Source: CAD feature listing. Evaluate the final solid. Frame: model axes, mm. Give positions to 0.01 mm unless a question says otherwise; leave off trailing zeros. Loops run counter-clockwise (first coordinate to the right, second up) from the corner with the lowest first, then second, coordinate; pieces in that order, holes last. Notation, with made-up numbers: (-39.5, 35.25) -> (-30.5, 35.25) arc R33 cw to (-30.5, 71.25) -> close; hole circle Ø5 at (84, -29.75). An arc over 180 degrees is marked (long way). Return JSON: item names as keys, results as strings. Group by question number.
(1) Cut plane C-C on z = -23. Return loops of the section in (x, y), then the cut area to 3 significant figures.
(2) Ray query, line 1 (X direction, y = 3.5, z = -107); line 2 (X direction, y = 0.5, z = 9). Return the intervals inside material, ascending. Write a range as from..to.
(3) Cut plane B-B on y = 0.5. Give the number of separate pieces and of enclosed holes in the cut face, then the cut area to 3 significant figures.
(4) Cut plane A-A on z = 104.5. Return loops of the section in (x, y).
(5) Pin query (flat end, axial travel): pin 1 (2.5 mm diameter, centred on x = -520, y = 0.5, fed in from -Z); pin 2 (2.5 mm diameter, centred on y = -0.5, z = -11, fed in from +X); pin 3 (2.5 mm diameter, centred on x = 528, y = 1, fed in from +Z). Return the tip coordinate at first contact, or that it passes through.
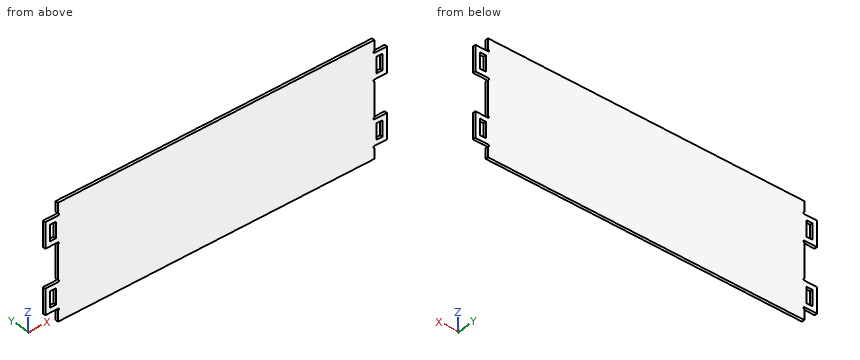
```python
from build123d import *

# Parameters (mm, degrees)
SKETCH1_W           = 18
SKETCH1_H           = 50
BOSS_EXTRUDE1_DEPTH = 4.3


with BuildPart() as part:
    # Sketch1 → Boss-Extrude1 (new body, symmetric)
    with BuildSketch(Plane(origin=(0, 0, 0), x_dir=(1, 0, 0), z_dir=(0, 1, 0))):
        with BuildLine():
            Line((-500, 179), (500, 179))
            Line((500, 179), (500, 146.36))
            ThreePointArc((500, 146.36), (496.82, 143.18), (500, 140))
            Line((500, 140), (540, 140))
            Line((540, 140), (540, 60))
            Line((540, 60), (500, 60))
            ThreePointArc((500, 60), (497, 57), (500, 54))
            Line((500, 54), (500, -54))
            ThreePointArc((500, -54), (497, -57), (500, -60))
            Line((500, -60), (540, -60))
            Line((540, -60), (540, -140))
            Line((540, -140), (500, -140))
            ThreePointArc((500, -140), (496.82, -143.18), (500, -146.36))
            Line((500, -146.36), (500, -179))
            Line((500, -179), (-500, -179))
            Line((-500, -179), (-500, -146.36))
            ThreePointArc((-500, -146.36), (-496.82, -143.18), (-500, -140))
            Line((-500, -140), (-540, -140))
            Line((-540, -140), (-540, -60))
            Line((-540, -60), (-500, -60))
            ThreePointArc((-500, -60), (-497, -57), (-500, -54))
            Line((-500, -54), (-500, 54))
            ThreePointArc((-500, 54), (-497, 57), (-500, 60))
            Line((-500, 60), (-540, 60))
            Line((-540, 60), (-540, 140))
            Line((-540, 140), (-500, 140))
            ThreePointArc((-500, 140), (-496.82, 143.18), (-500, 146.36))
            Line((-500, 146.36), (-500, 179))
        make_face()
        with Locations((-516, 100)):
            Rectangle(SKETCH1_W, SKETCH1_H, mode=Mode.SUBTRACT)
        with Locations((-516, -100)):
            Rectangle(SKETCH1_W, SKETCH1_H, mode=Mode.SUBTRACT)
        with Locations((516, -100)):
            Rectangle(SKETCH1_W, SKETCH1_H, mode=Mode.SUBTRACT)
        with Locations((516, 100)):
            Rectangle(SKETCH1_W, SKETCH1_H, mode=Mode.SUBTRACT)
    extrude(amount=BOSS_EXTRUDE1_DEPTH, both=True)


solid = part.part
```
Answers:
{
 "1": {"outline": "(-500, -4.3) -> (500, -4.3) -> (500, 4.3) -> (-500, 4.3) -> close", "area": "8,600 mm²"},
 "2": {"line 1": "-540..-525, -507..507, 525..540", "line 2": "-500..500"},
 "3": {"separate pieces": "1", "enclosed holes": "4", "area": "367,000 mm²"},
 "4": {"outline": "(-540, -4.3) -> (-525, -4.3) -> (-525, 4.3) -> (-540, 4.3) -> close; (-507, -4.3) -> (507, -4.3) -> (507, 4.3) -> (-507, 4.3) -> close; (525, -4.3) -> (540, -4.3) -> (540, 4.3) -> (525, 4.3) -> close"},
 "5": {"pin 1": "z = -140", "pin 2": "x = 500", "pin 3": "z = 140"}
}
